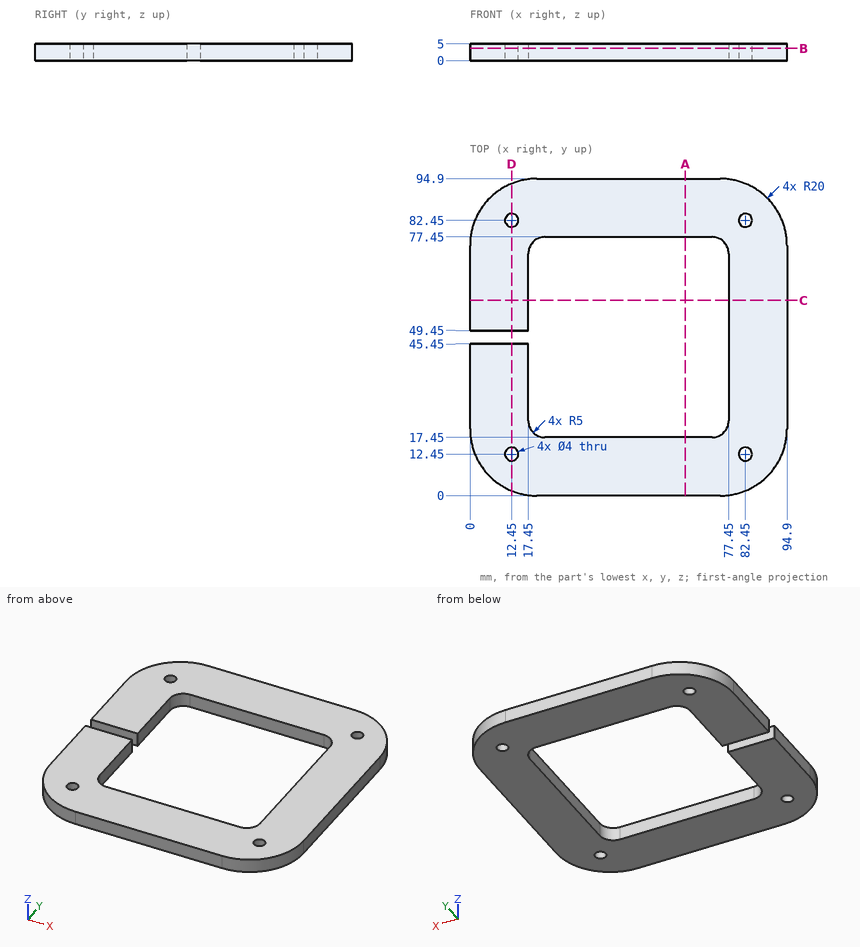
Study the drawing (mm; zero at the part's minimum x, y, z) and answer. Give positions to 0.01 mm unless a question says otherwise; leave off trailing zeros. Loops run counter-clockwise (first coordinate to the right, second up) from the corner with the lowest first, then second, coordinate; pieces in that order, holes last. Notation, with made-up numbers: (39, 10.5) - (91, 10.5) arc R22 ccw to (91, 30.5) - close; hole circle Ø9 at (-9.5, 28). An arc over 180 degrees is marked (long way). Use CSV: the item, a comma, the result in double quotes. Start each with the question number.
(1) Find section D-D, the plane x = 12.45. Determine the outline of the cut face in (y, z).
(2) Each of these flat-tipped pins is pushed along its axis until it touches: pin 1 (1.5 mm diameter, centred on x = 13, z = 3.5, fed in from +Y); pin 2 (2.5 mm diameter, centred on x = 82.45, y = 82.45, fed in from -Z); pin 3 (3 mm diameter, centred on x = 10.5, z = 3, fed in from -Y); pin 4 (3 mm diameter, centred on x = 12.5, z = 2, fed in from +Y). Where does it stop, or does it pass through?
(3) Find section A-A, the plane x = 64.5. Determine the outline of the cut face in (y, z), plus the area to 4 significant figures.
(4) Find the intervals of material crossed by L1, parallel to Y at x = 51.5, z = 2.2; L2, parallel to Y at x = 12.45, z = 3.1, in increasing order.
(5) Find section B-B, the plane z = 3.7. Determine the outline of the cut face in (x, y), plus the area to 3 significant figures.
Results found:
1,outline,"(1.48, 0) - (10.45, 0) - (10.45, 5) - (1.48, 5) - close; (14.45, 0) - (45.45, 0) - (45.45, 5) - (14.45, 5) - close; (49.45, 0) - (80.45, 0) - (80.45, 5) - (49.45, 5) - close; (84.45, 0) - (93.42, 0) - (93.42, 5) - (84.45, 5) - close"
2,pin 1,"y = 93.9"
2,pin 2,"through"
2,pin 3,"y = 1.67"
2,pin 4,"y = 93.98"
3,outline,"(0, 0) - (17.45, 0) - (17.45, 5) - (0, 5) - close; (77.45, 0) - (94.9, 0) - (94.9, 5) - (77.45, 5) - close"
3,area,"174.5 mm^2"
4,L1,"0 to 17.45, 77.45 to 94.9"
4,L2,"1.48 to 10.45, 14.45 to 45.45, 49.45 to 80.45, 84.45 to 93.42"
5,outline,"(0, 20) arc R20 ccw to (20, 0) - (74.9, 0) arc R20 ccw to (94.9, 20) - (94.9, 74.9) arc R20 ccw to (74.9, 94.9) - (20, 94.9) arc R20 ccw to (0, 74.9) - (0, 49.45) - (17.45, 49.45) - (17.45, 72.45) arc R5 cw to (22.45, 77.45) - (72.45, 77.45) arc R5 cw to (77.45, 72.45) - (77.45, 22.45) arc R5 cw to (72.45, 17.45) - (22.45, 17.45) arc R5 cw to (17.45, 22.45) - (17.45, 45.45) - (0, 45.45) - close; hole circle Ø4 at (12.45, 12.45); hole circle Ø4 at (12.45, 82.45); hole circle Ø4 at (82.45, 12.45); hole circle Ø4 at (82.45, 82.45)"
5,area,"4,960 mm^2"
